The model under review builds one solid part; all positions refer to its coordinate system, in mm. A direction names the side the tool comes from. Coordinates: 2 decimals unless noted, no trailing zeros. Order: outer loops, then holes, each group sorted by start corner. A loop starts at its lowest first (then second) coordinate and runs counter-clockwise, first axis right, second up. Notation, with made-up numbers: M 84,81 L 88,81 A22 ccw 88,95 Z; hole C 35,13.5 d5. An arc over 180 degrees is marked long. Answer as CSV lines item,"result". Start each with the question number.
Q1. Consider section A-A on y = -4.5. Write out the cut boundary in (x, z).
Q2. Consider section C-C on z = 48. Write out the cut boundary in (x, y).
Q3. Machinability: for faces 5 (the face through (18, -3, -15)), 6 (the face through (-19, -12.5, -1)), 7 (the face through (18, 4, 13)), 8 (the face through (0, -2.5, 57)), which of the approach directions +Z, -Z, +X, -X, +Y, -Y give a long, thin tool a straight path to every point of the face, cutting with its end or side? Answer none if there is none.
Q4. The part is to be moulded in two halves that separate along Z. For faces 1 (the face through (-0.3, -5.4, 58.5)), 2 (the face through (19, -12.5, -1)), 3 (the face through (0.25, -1.16, -0.17)), 4 (the face through (0, -6, 56)), say which applies: +Z half, -Z half, draft (parallel to the pull), parting line (faces both ways), or undercut.
Q5. Wall thickness on L1, parallel to X at y = -0.5, z = -54.5; L2, parallel to Y at x = -4.5, z = 5.5; L3, parallel to Y at x = 12, z = -53: over which ranges is each line inside the solid? List them lowest first. Write a range as [from, to].
Q6. For P1, Ø1.5, axis at x = 4, z = -28.5, coming from the +Y side; P2, Ø2, axis at x = -1, z = 57.5, coming from the +Y side; P3, Ø1, axis at x = 10, z = 14, coming from the -Y side; P4, Ø8, axis at x = 15.5, y = 7, coming from the -Z side, all flat-tipped, find the tip position at first contact; note any pin that passes through.
Q7. Consider section D-D on y = 2. Write out the cut boundary in (x, z).
Q8. Consider section B-B on x = -7.5. Write out the cut boundary in (y, z).
from build123d import *

# Parameters (mm, degrees)
SKETCH1_W           = 40
SKETCH1_H           = 25
BOSS_EXTRUDE1_DEPTH = 60
CUT_EXTRUDE3_DEPTH  = 18
SKETCH6_W           = 36
SKETCH6_H           = 8
BOSS_EXTRUDE2_DEPTH = 4
SKETCH7_R           = 500
SKETCH7_R_2         = 101.5
CUT_EXTRUDE4_DEPTH  = 26


with BuildPart() as part:
    # Sketch1 → Boss-Extrude1 (new body, symmetric)
    with BuildSketch(Plane.XY):
        Rectangle(SKETCH1_W, SKETCH1_H)
    extrude(amount=BOSS_EXTRUDE1_DEPTH, both=True)

    # Sketch4 → Cut-Extrude3 (cut, symmetric)
    with BuildSketch(Plane(origin=(0, 0, 0), x_dir=(0, 0, -1), z_dir=(1, 0, 0))):
        Polygon((-60, -10.5), (58, 12.5), (-60, 12.5), align=None)
        Polygon((-58, -12.5), (60, 10.5), (60, -12.5), align=None)
    extrude(amount=CUT_EXTRUDE3_DEPTH, both=True, mode=Mode.SUBTRACT)

    # Sketch6 → Boss-Extrude2 (add)
    with BuildSketch(Plane.XY.offset(60)):
        with Locations((0, -6.5)):
            Rectangle(SKETCH6_W, SKETCH6_H)
    extrude(amount=-BOSS_EXTRUDE2_DEPTH)

    # Sketch7 → Cut-Extrude4 (cut, through all)
    with BuildSketch(Plane(origin=(0, 12.5, 0), x_dir=(1, 0, 0), z_dir=(0, 1, 0))):
        with Locations((0, 43)):
            Circle(SKETCH7_R)
        with Locations((0, 43)):
            Circle(SKETCH7_R_2, mode=Mode.SUBTRACT)
    extrude(amount=-CUT_EXTRUDE4_DEPTH, mode=Mode.SUBTRACT)


solid = part.part
Evaluation:
1,outline,"M -20,-60 L -18,-60 L -18,16.96 L 18,16.96 L 18,-60 L 20,-60 L 20,56.51 A101.5 ccw -20,56.51 Z; hole M -18,29.22 L 18,29.22 L 18,56 L -18,56 Z"
2,outline,"M -20,-12.5 L -18,-12.5 L -18,-10.55 L 18,-10.55 L 18,-12.5 L 20,-12.5 L 20,12.5 L 18,12.5 L 18,-8.16 L -18,-8.16 L -18,12.5 L -20,12.5 Z"
3,face 5,"-Z, -Y"
3,face 6,"+Z, -Z, +X, -X, -Y"
3,face 7,"+Y"
3,face 8,"+Z, +Y"
4,face 1,"+Z half"
4,face 2,"draft"
4,face 3,"-Z half"
4,face 4,"undercut"
5,L1,"x = [-20, -18], [18, 20]"
5,L2,"y = [-2.27, 0.12]"
5,L3,"y = [9.14, 11.53]"
6,P1,"stops at y = 6.9"
6,P2,"stops at y = -2.5"
6,P3,"stops at y = -4.02"
6,P4,"stops at z = -60"
7,outline,"M -20,-60 L -18,-60 L -18,-16.39 L 18,-16.39 L 18,-60 L 20,-60 L 20,56.51 A101.5 ccw 18,56.89 L 18,-4.13 L -18,-4.13 L -18,56.89 A101.5 ccw -20,56.51 Z"
8,outline,"M -12.5,58 L 10.5,-60 L 12.5,-60 L 12.5,-58 L -9.72,56 L -2.5,56 L -2.5,58.22 L -12.5,58.22 Z"
